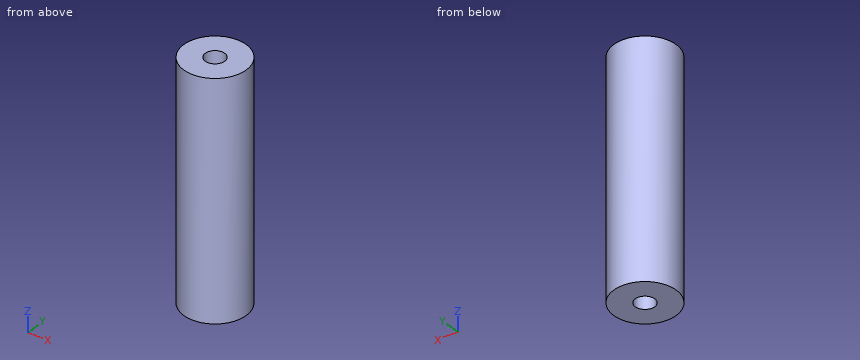
```python
from build123d import *

# Parameters (mm, degrees)
SKETCH1_R           = 4
BOSS_EXTRUDE1_DEPTH = 15


with BuildPart() as part:
    # Sketch1 → Boss-Extrude1 (new, symmetric)
    with BuildSketch(Plane.XY):
        Circle(SKETCH1_R)
    extrude(amount=BOSS_EXTRUDE1_DEPTH, both=True)

    # Sketch3 → M3 Tapped Hole1 (revolve, cut)
    with BuildSketch(Plane(origin=(0, 0, 15), x_dir=(0, -1, 0), z_dir=(1, 0, 0))):
        Polygon((0, 0), (0, 8.251075774), (1.25, 7.5), (1.25, 0), align=None)
    m3_tapped_hole1 = revolve(axis=Axis((0, 0, 21.35), (0, 0, -1)), mode=Mode.SUBTRACT)

    # Mirror1: M3 Tapped Hole1 across plane
    add(m3_tapped_hole1.mirror(Plane.XY), mode=Mode.SUBTRACT)


solid = part.part
```
Verification items for the finished model (mm, model axes). Round coordinates to 2 decimals unless told otherwise and drop trailing zeros. Write each loop counter-clockwise with the first axis right and the second up, starting at its lowest first coordinate (ties: lowest second). Pieces come first, ordered by that corner, then holes. Notation, with made-up numbers: (46, 41) -> (97, 41) arc R21 cw to (97, 45) -> close; hole circle Ø7 at (15.25, -32.5). An arc over 180 degrees is marked (long way). Write each question's results on one line, items separated by ' | '. Start each with the question number.
1. Depth check by flat-ended pin: P1, Ø1.5, axis at x = 0, y = 0, coming from the +Z side; P2, Ø1, axis at x = 2.5, z = -11.5, coming from the +Y side. Enter the tip coordinate at first touch or a pass-through.
2. Cross-section at A-A (z = 12.5). Enter the section's corners in (x, y).
3. Cross-section at C-C (x = -2). Enter the section's corners in (y, z), then the cut area to 3 significant figures.
4. Cross-section at B-B (z = 3.75). Enter the section's corners in (x, y).
5. Material ranges on probe 1 along Y at (x, z) = (0, -12); probe 2 along Y at (x, z) = (-0.5, 13.5); probe 3 along Y at (x, z) = (-2, -12), recorded low to high. Write a range as from..to.
Solutions:
1) P1: stops at z = 7.2 | P2: stops at y = 3.46
2) outline: circle Ø8 at (0, 0); hole circle Ø2.5 at (0, 0)
3) outline: (-3.46, -15) -> (3.46, -15) -> (3.46, 15) -> (-3.46, 15) -> close | area: 208 mm2
4) outline: circle Ø8 at (0, 0)
5) probe 1: y = -4..-1.25, 1.25..4 | probe 2: y = -3.97..-1.15, 1.15..3.97 | probe 3: y = -3.46..3.46
